Autodesk Inventor part; units mm, degrees
ref_plane "Start Plane" through (0, 0, 20) normal (0, 0, 1) x (1, 0, 0)
ref_plane "End Plane" through (0, 0, 167.2955) normal (0, 0, 1) x (1, 0, 0)
ref_plane "Work Plane4" through (0, -20.6823, 167.9321) normal (0, 0.6823, 0.7311) x (1, 0, 0)
ref_plane "Start Plane" through (0, 0, 20) normal (0, 0, 1) x (1, 0, 0)
ref_plane "End Plane" through (0, 0, 167.2955) normal (0, 0, 1) x (1, 0, 0)
sketch "Sketch" plane through (0, 0, 0) normal (0, 0, 1) x (1, 0, 0)
  line L0 (-20, -12) -> (-20, 12)
  line L1 (-12, 20) -> (12, 20)
  line L2 (20, 12) -> (20, -12)
  line L3 (12, -20) -> (-12, -20)
  arc A0 (-20, -12) -> (-12, -20) centre (-12, -12) ccw
  arc A1 (20, 12) -> (12, 20) centre (12, 12) ccw
  arc A2 (-12, 20) -> (-20, 12) centre (-12, 12) ccw
  arc A3 (12, -20) -> (20, -12) centre (12, -12) ccw
  arc A4 (-12, 16) -> (-16, 12) centre (-12, 12) ccw
  line L4 (-12, 16) -> (12, 16)
  arc A5 (16, 12) -> (12, 16) centre (12, 12) ccw
  line L5 (16, 12) -> (16, -12)
  arc A6 (12, -16) -> (16, -12) centre (12, -12) ccw
  line L6 (12, -16) -> (-12, -16)
  arc A7 (-16, -12) -> (-12, -16) centre (-12, -12) ccw
  line L7 (-16, -12) -> (-16, 12)
  line L8 (0, 30.3196) -> (0, -30.3196) construction
  line L9 (-30.3196, 0) -> (30.3196, 0) construction
  dimension "d7" = 8
  dimension "d9" = 40
  dimension "d11" = 40
  dimension "d12" = 4
  dimension "d15" = 20
  dimension "d16" = 20
extrude "Body" add sketch "Sketch" along normal up to surface (147.2955 mm away) from surface at 20
sketch "Sketch3" plane through (0, 0, 0) normal (0, 0, 1) x (1, 0, 0)
  line L0 (0, 0) -> (10, 0)
ref_plane "Work Plane3" through (0, 0, 0) normal (0, -1, 0) x (1, 0, 0)
ref_plane "Work Plane4" through (0, -20.6823, 167.9321) normal (0, 0.6823, 0.7311) x (1, 0, 0)
split "Split1" plane through (0, -20.6823, 167.9321) removes the side toward (0, 0.6823, 0.7311)
ref_plane "Work Plane5" through (-12, 6500, 20) normal (0, 0, -1) x (-1, 0, 0)
split "Split2" plane through (-12, 6500, 20) removes the side toward (0, 0, -1)
sketch "Sketch4" plane through (0, 0, 0) normal (0, -1, 0) x (1, 0, 0)
  line L0 (-2, 20) -> (12, 20)
  line L1 (-2, 167.2955) -> (12, 167.2955)
  dimension "d18" = 147.2955
equation "\"d7\" = G_IR"
equation "\"d9\" = G_W"
equation "\"d11\" = G_H"
equation "\"d12\" = G_T"
equation "\"d15\" = 0.5 * d9"
equation "\"d16\" = 0.5 * d11"
equation "\"d3\" = G_L"
equation "\"G_W\" = 40"
equation "\"G_H\" = 40"
equation "\"G_T\" = 4"
equation "\"G_IR\" = 8"
equation "\"G_L\" = d18"
equation "\"G_OFFSET_END\" = 17.29549"
equation "\"d14\" = G_OFFSET_END + B_L"
properties part number "ISO 10799-2 - 40x40x4 - 147,3" material "Steel, Mild"
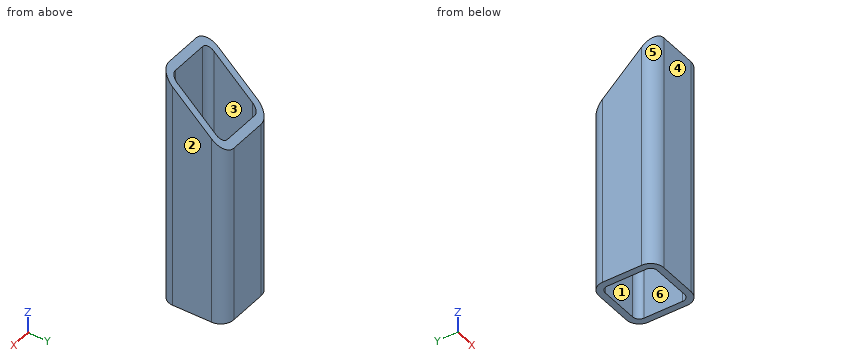
Verification items for the finished model (mm, model axes). Face numbers are marked on the shaded views. A direction names the side the tool comes from. Coordinates: 2 decimals unless noted, no trailing zeros. Order: outer loops, then holes, each group sorted by start corner. A loop starts at its lowest first (then second) coordinate and runs counter-clockwise, first axis right, second up. Notation, with made-up numbers: (71, 2) -> (95, 2) arc R6 cw to (95, 7) -> close; hole circle Ø7 at (72, 7.5). An arc over 180 degrees is marked (long way). Answer as CSV lines item,"result". Start each with the question number.
1) Gauge pin test, flat ends, axial feed: pin 1 Ø1 at (x, z) = (-13, 143) entering from +Y; pin 2 Ø1 at (y, z) = (13, 58.5) entering from -X; pin 3 Ø12 at (x, y) = (-8, 14.5) entering from +Z. Record the tip position at first contact, or that the pin passes through.
2) Cross-section at A-A, the plane x = 7. Record the boundary of the cut face in (y, z), then the cut area to 3 significant figures.
3) Release check for a two-part mould opening along X. For the marked faces 1, 2, 3 and 4 record: released by +X, released by -X, zero draft, split by the parting line, or undercut.
4) Material ranges on L1, parallel to Y at x = -8, z = 84; L2, parallel to Y at x = -7.5, z = 160.5, recorded low to high. Write a range as [from, to].
5) Cross-section at B-B, the plane z = 37. Record the boundary of the cut face in (x, y), then the cut area to 3 significant figures.
6) Cross-section at C-C, the plane y = -7.5. Record the boundary of the cut face in (x, z).
7) Set-up check for the marked faces 5 and 6: record each of +Z, -Z, +X, -X, +Y, -Y from which the full face is reachable in a straight line by a thin tool's end or side.
8) Cross-section at D-D, the plane z = 142. Record the boundary of the cut face in (x, y), then the cut area to 3 significant figures.
Conclusion:
1,pin 1,"stops at y = -15.71"
1,pin 2,"stops at x = -19.98"
1,pin 3,"stops at z = 134.15"
2,outline,"(-20, 20) -> (-16, 20) -> (-16, 163.56) -> (-20, 167.3) -> close; (16, 20) -> (20, 20) -> (20, 129.97) -> (16, 133.7) -> close"
2,area,"1,030 mm²"
3,face 1,"undercut"
3,face 2,"released by +X"
3,face 3,"undercut"
3,face 4,"zero draft"
4,L1,"y = [-20, -16], [16, 20]"
4,L2,"y = [-20, -16]"
5,outline,"(-20, -12) arc R8 ccw to (-12, -20) -> (12, -20) arc R8 ccw to (20, -12) -> (20, 12) arc R8 ccw to (12, 20) -> (-12, 20) arc R8 ccw to (-20, 12) -> close; hole (-16, -12) arc R4 ccw to (-12, -16) -> (12, -16) arc R4 ccw to (16, -12) -> (16, 12) arc R4 ccw to (12, 16) -> (-12, 16) arc R4 ccw to (-16, 12) -> close"
5,area,"535 mm²"
6,outline,"(-20, 20) -> (-16, 20) -> (-16, 155.63) -> (-20, 155.63) -> close; (16, 20) -> (20, 20) -> (20, 155.63) -> (16, 155.63) -> close"
7,face 5,"+Z, -Z, -X, -Y"
7,face 6,"+Z, -Z"
8,outline,"(-20, -12) arc R8 ccw to (-12, -20) -> (12, -20) arc R8 ccw to (20, -12) -> (20, 7.1) -> (16, 7.1) -> (16, -12) arc R4 cw to (12, -16) -> (-12, -16) arc R4 cw to (-16, -12) -> (-16, 7.1) -> (-20, 7.1) -> close"
8,area,"324 mm²"
